Can you work these out from the drawing? Everything is in mm from the part's minimum corner. Coordinates: 2 decimals unless noted, no trailing zeros. Order: outer loops, then holes, each group sorted by start corner. A loop starts at its lowest first (then second) coordinate and runs counter-clockwise, first axis right, second up. Notation, with made-up numbers: (46, 76.25) -> (99, 76.25) arc R14 ccw to (99, 86.25) -> close; hole circle Ø3 at (-33, 69). An arc over 180 degrees is marked (long way). Put each result on its own line as item: value. Start each with the question number.
Q1. Please list where these lines run through material, in increasing order: line 1 along X through (y, z) = (5.75, 85) (1 decimal); line 2 along X through (y, z) = (2.5, 69); line 3 along Z through (x, y) = (74.5, 4.5) (1 decimal).
Q2. If we section it at A-A (z = 101): Count the separate pieces of the cut face and the enclosed holes in it.
Q3. Will these pins go through, and if not, where does the flat tip stop? pin 1 (8.5 mm diameter, centred on x = 29.37, z = 138.97, fed in from -Y); pin 2 (2 mm diameter, centred on x = 147.5, y = 5, fed in from +Z) (1 decimal); pin 3 (1.9 mm diameter, centred on x = 42, y = 2, fed in from +Z); pin 4 (1.9 mm diameter, centred on y = 2.5, z = 91.5, fed in from +X).
Q4. If we section it at D-D (z = 152.5): Please give me the cut outline in (x, y).
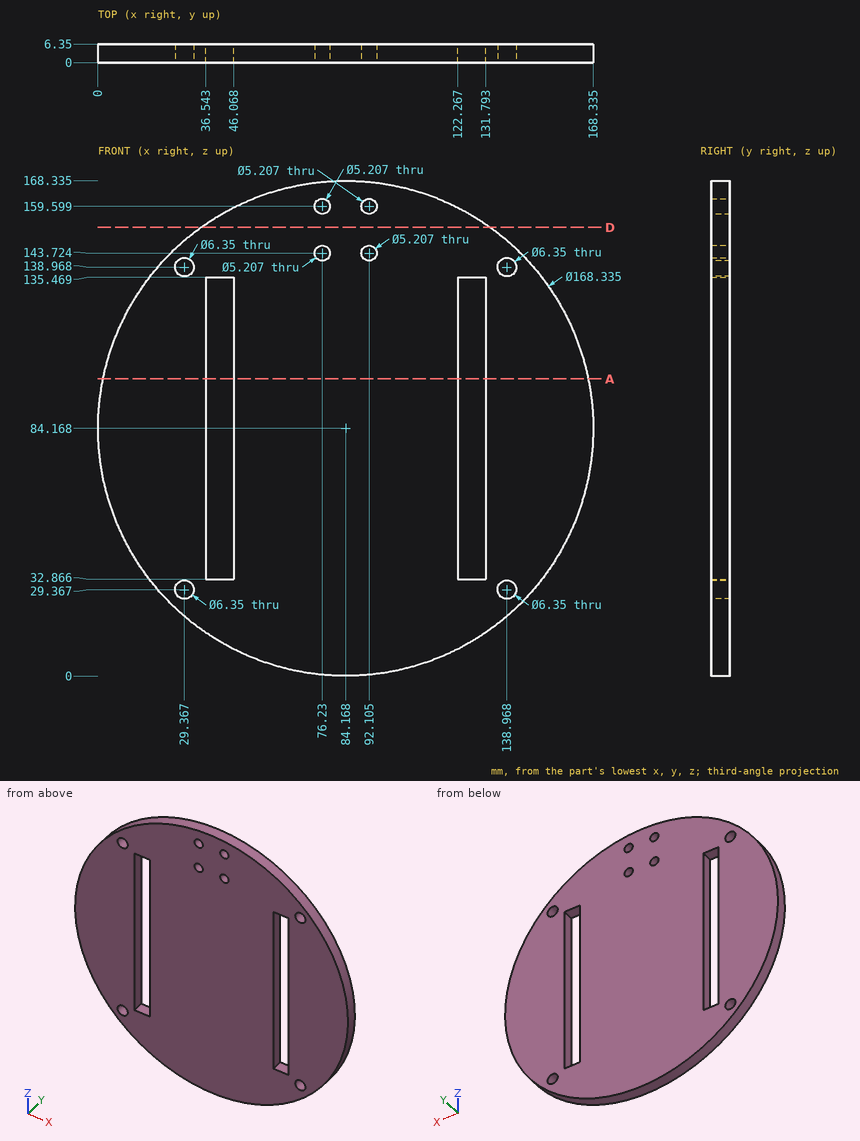
The answers:
1. line 1: 0 to 36.5, 46.1 to 122.3, 131.8 to 168.3
1. line 2: 1.38 to 36.54, 46.07 to 122.27, 131.79 to 166.96
1. line 3: 0.6 to 141.8, 145.7 to 157.7, 161.5 to 167.8
2. separate pieces: 3
2. enclosed holes: 0
3. pin 1: y = 0
3. pin 2: z = 140.7
3. pin 3: z = 157.55
3. pin 4: x = 168.09
4. outline: (35.03, 0) -> (133.31, 0) -> (133.31, 6.35) -> (35.03, 6.35) -> close
